The listing builds one solid part. Answer for the finished solid, in the listing's coordinates (mm). Face numbers are marked on the shaded views. A direction names the side the tool comes from. Coordinates: 2 decimals unless noted, no trailing zeros. Order: outer loops, then holes, each group sorted by start corner. A loop starts at its lowest first (then second) coordinate and runs counter-clockwise, first axis right, second up. Notation, with made-up numbers: (63, -11) -> (69, -11) arc R11 ccw to (69, -2) -> close; hole circle Ø7 at (61.5, 31). An arc over 180 degrees is marked (long way). Put each result on its own line as item: value. Start each with the question number.
```python
from build123d import *

# Parameters (mm, degrees)
F2_T = -1
F3_R = 5
F4_R = 5


with BuildPart() as f1:
    # F0 (on Front) → F1 (revolve)
    with BuildSketch(Plane.XZ):
        Polygon((0, 100.964410305), (-30, 100.964410305), (-48.0997800827, 20.2851913869), (-43.2369445397, 0), (-31.5237879753, -14.6114934236), (-3.8748302031, -23.7388100573), (0, -25.0179469585), align=None)
        Polygon((0, -69.035589695), (0, -25.0179469585), (-3.8748302031, -23.7388100573), (-3.8748302031, -58.9307323098), (-36.4315584302, -69.035589695), align=None)
    revolve(axis=Axis((0, 0, 15.964410305), (0, 0, -1)))

    # F2
    f2_openings = [f1.faces().sort_by_distance(p)[0] for p in [
        (0, 0, 100.96441),
    ]]
    offset(amount=F2_T, openings=f2_openings, kind=Kind.INTERSECTION)

    # F3
    f3_edges = [f1.edges().sort_by_distance(p)[0] for p in [
        (3.87483, 0, -58.930732),
        (3.87483, 0, -23.73881),
    ]]
    fillet(f3_edges, radius=F3_R)

    # F4
    f4_edges = [f1.edges().sort_by_distance(p)[0] for p in [
        (31.523788, 0, -14.611493),
    ]]
    fillet(f4_edges, radius=F4_R)


solid = f1.part
```
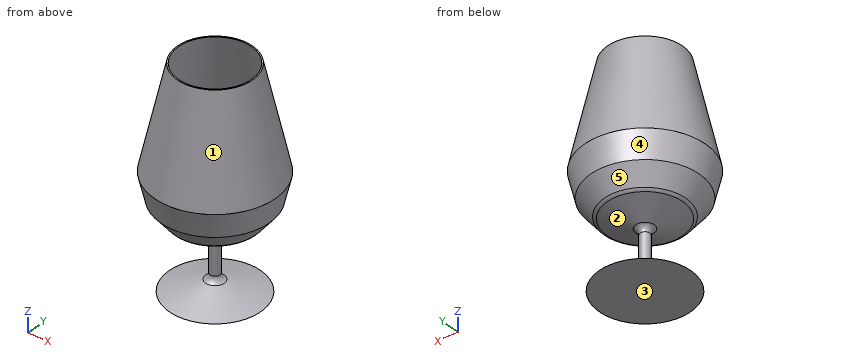
(1) The part is cut by section A-A on y = 21. Count the separate pieces of the cut face and the enclosed holes in it, plus the area to 3 significant figures.
(2) A tool of negligible diameter and unlimited length cuts with its end or side. For the marked faces 4 and 5, from which of +Z, -Z, +X, -X, +Y, -Y can it reach the whole face along a straight path? Write none if from no direction.
(3) The part is cut by section C-C on z = -3.5. Determine the outline of the cut face in (x, y).
(4) Find the intervals of material crossed by L1, parallel to X at y = 0, z = -32; L2, parallel to Z at x = -14, y = 25, in increasing order.
(5) Each of these flat-tipped pins is pushed along its axis until it touches: P1, Ø1, axis at y = -6.5, z = -12, coming from the -X side; P2, Ø5, axis at x = 7, z = 77, coming from the -Y side; P3, Ø6.5, axis at x = 0, y = 0, coming from the +Z side. Where does it stop, or does it pass through?
(6) The part is cut by section D-D on z = 14. Determine the outline of the cut face in (x, y), plus the area to 3 significant figures.
(7) For a pull along Z with two mould halves and no side action, classify the marked faces 1, 2 and 3 as released by +Z, released by -Z, zero draft, split by the parting line, or undercut.
Worked out:
1. separate pieces: 2
1. enclosed holes: 1
1. area: 446 mm2
2. face 4: -Z
2. face 5: none
3. outline: circle Ø80.86 at (0, 0); hole circle Ø78.3 at (0, 0)
4. L1: -3.87 to -2.87, 2.87 to 3.87
4. L2: -69.04 to -68.04, -67.67 to -66.62, -15.56 to -14.51
5. P1: x = -33.4
5. P2: y = -35.4
5. P3: z = -22.89
6. outline: circle Ø93.19 at (0, 0); hole circle Ø91.13 at (0, 0)
6. area: 298 mm2
7. face 1: released by +Z
7. face 2: undercut
7. face 3: released by -Z
